Source: CAD feature listing. Evaluate the final solid. Frame: model axes, mm. A direction names the side the tool comes from. Coordinates: 2 decimals unless noted, no trailing zeros. Loops run counter-clockwise (first coordinate to the right, second up) from the corner with the lowest first, then second, coordinate; pieces in that order, holes last. Notation, with made-up numbers: (23.5, -25.5) - (28.5, -25.5) arc R20 ccw to (28.5, -8.5) - close; hole circle Ø7 at (-23, 82). An arc over 180 degrees is marked (long way). Write item = value, one per line. Start each with the question number.
Autodesk Inventor part; units mm, degrees
ref_plane "YZ Plane" through (0, 0, 0) normal (1, 0, 0) x (0, 1, 0)
ref_plane "XZ Plane" through (0, 0, 0) normal (0, 1, 0) x (-1, 0, 0)
ref_plane "XY Plane" through (0, 0, 0) normal (0, 0, 1) x (1, 0, 0)
sketch "Sketch1" plane through (0, 0, 0) normal (0, 0, 1) x (1, 0, 0)
  line L0 (65.359, 13) -> (101.145, 9.0808) construction
  circle A0 centre (65.359, 13) radius 3 construction
  circle A1 centre (65.359, 13) radius 4.025
  circle A2 centre (65.359, 13) radius 7
  arc A3 (103.9065, 14.4076) -> (101.5853, 15.5481) centre (76.292, -38.8601) ccw construction
  arc A4 (98.0987, 3.9117) -> (67.8539, 6.4597) centre (80.3286, -26.2417) ccw
  circle A5 centre (101.145, 9.0808) radius 2.5 construction
  circle A6 centre (101.145, 9.0808) radius 3.525
  circle A7 centre (101.145, 9.0808) radius 6
  line L1 (101.145, 9.0808) -> (116.8532, -6.3223) construction
  circle A8 centre (116.8532, -6.3223) radius 10 construction
  circle A9 centre (116.8532, -6.3223) radius 7.025 construction
  line L2 (104.4969, 14.0572) -> (122.4397, 1.9718) construction
  line L3 (96.2353, 5.6319) -> (108.6703, -12.0703) construction
  line L4 (121.8748, 2.4728) -> (123.0794, 1.6615) construction
  arc A10 (101.4998, 3.0913) -> (116.7565, 8.3414) centre (99.726, 33.0388) ccw
  arc A11 (116.4477, 11.8091) -> (81.0555, 20.9505) centre (72.64, -84.7149) ccw
  arc A12 (116.7565, 8.3414) -> (116.4477, 11.8091) centre (115.6212, 9.9879) ccw
  line L5 (65.359, 13) -> (100, 0) construction
  arc A13 (112.7035, 13.4223) -> (110.8303, 9.9119) centre (111.9476, 11.5707) ccw
  line L6 (101.145, 9.0808) -> (80.4889, 1.5095) construction
  circle A14 centre (80.4889, 1.5095) radius 7.025 construction
  circle A15 centre (80.4889, 1.5095) radius 10 construction
  line L7 (110.8303, 9.9119) -> (114.9091, 7.1646)
  arc A16 (81.0555, 20.9505) -> (63.915, 19.8494) centre (76.292, -38.8601) ccw
  arc A17 (101.5853, 15.5481) -> (81.0555, 20.9505) centre (76.292, -38.8601) ccw construction
  line L8 (78.8119, 11.3678) -> (100.1388, 14.9958) construction
  line L9 (78.7951, 11.4664) -> (105.6086, 16.0277)
  arc A18 (78.7951, 11.4664) -> (72.6773, 7.9118) centre (80.4889, 1.5095) ccw
  point P0 (0, 0)
  point P1 (104.5045, 16.3824)
  dimension "d57" = 20
  dimension "d1" = 8.05
  dimension "d2" = 6
  dimension "d3" = 14
  dimension "d4" = 60
  dimension "d5" = 35
  dimension "d8" = 22
  dimension "d10" = 12
  dimension "d11" = 7.05
  dimension "d12" = 20
  dimension "d13" = 14.05
  dimension "d15" = 0.1
  dimension "d16" = 30
  dimension "d17" = 5
  dimension "d18" = 2
  dimension "d19" = 106
  dimension "d21" = 121
  dimension "d46" = 13
  dimension "d47" = 37
  dimension "d48" = 18
  dimension "d50" = 0
  dimension "d51" = 100
  dimension "d53" = 2
  dimension "d54" = 4
  dimension "d55" = 22
  dimension "d56" = 14.05
  dimension "d65" = 14.32
  dimension "d68" = 26.38
  dimension "d69" = 0.1
  dimension "d70" = 0.1
  dimension "d72" = 36
extrude "Extrusion5" add sketch "Sketch1" against normal blind 3 contours A2 | A2 A16 A11 L9 A18 A4 | A11 A12 A10 L7 A13
extrude "Extrusion6" add sketch "Sketch1" against normal blind 1.8 contours A18 L9 A11 A13 L7 A10 A7 A4 | A7
properties part number "揺動節" material "Aluminum 2014-T6"
Item 1: Cut plane C-C (z = -0.55). State how many separate pieces and enclosed holes the cut face has, then the cut area to 3 significant figures.
Item 2: Reachability of faces 4 (the flat face through (112.84, 8.56, -2.39)), 5 (the cylindrical face through (110.203, 12.548, -2.392)), 6 (the cylindrical face through (104.4, 7.73, -0.89)) from +Z, -Z, +X, -X, +Y, -Y: full face, straight path, thin tool, end or side. Return the list, or none.
Item 3: First-contact query: pin 1 (1 mm diameter, centred on x = 78.5, z = -0.5, fed in from -Y); pin 2 (10.5 mm diameter, centred on x = 65.359, y = 13, fed in from -Z); pin 3 (1.5 mm diameter, centred on x = 104.5, z = -2, fed in from +Y). Flat tips, straight axial feed; report the tip coordinate or a pass-through.
Item 4: Material intervals for L1, parallel to X at y = 10.75, z = -1.9; L2, parallel to Y at x = 65.5, z = -0.25; L3, parallel to Z at x = 89, y = 11.5, sorted ascending. Write a range as [from, to].
Item 5: Draft query along X for faces 1 (the cylindrical face through (72.566, 21.024, -1.479)), 2 (the flat face through (92.014, 13.715, -2.392)), 3 (the cylindrical face through (109.38, 4.634, -0.812)). Return one class per face: released by +X, released by -X, zero draft, split by the parting line, or undercut.
Item 6: Cut plane D-D (x = 86.5). Return the cut outline in (y, z), then the cut area to 3 significant figures.
Item 7: Cut plane B-B (x = 99). Return the cut outline in (y, z), then the cut area to 3 significant figures.
Item 8: Cut plane A-A (y = 15.25). Return the cut outline in (x, z), then the cut area to 3 significant figures.
Responses:
q1.separate_pieces = 1
q1.enclosed_holes = 2
q1.area = 610 mm2
q2.face_4 = -Z, -Y
q2.face_5 = -Z
q2.face_6 = +Z, -Z
q3.pin_1 = 8.68
q3.pin_2 = -3
q3.pin_3 = 16.62
q4.L1 = [58.73, 62.02], [68.7, 76.41], [110.12, 117.47]
q4.L2 = [6, 8.98], [17.02, 20.16]
q4.L3 = [-1.8, 0]
q5.face_1 = split by the parting line
q5.face_2 = undercut
q5.face_3 = released by +X
q6.outline = (8.21, -1.8) - (12.78, -1.8) - (12.78, -3) - (20.38, -3) - (20.38, 0) - (8.21, 0) - close
q6.area = 31.0 mm2
q7.outline = (3.48, -1.8) - (6.28, -1.8) - (6.28, 0) - (3.48, 0) - close; (11.88, -1.8) - (14.9, -1.8) - (14.9, -3) - (17.96, -3) - (17.96, 0) - (11.88, 0) - close
q7.area = 19.7 mm2
q8.outline = (58.73, -3) - (62.02, -3) - (62.02, 0) - (58.73, 0) - close; (68.7, -3) - (101.04, -3) - (101.04, -1.8) - (107.9, -1.8) - (107.9, 0) - (68.7, 0) - close
q8.area = 119 mm2
